The listing builds one solid part. Answer for the finished solid, in the listing's coordinates (mm). A direction names the side the tool comes from. Coordinates: 2 decimals unless noted, no trailing zeros. Loops run counter-clockwise (first coordinate to the right, second up) from the corner with the lowest first, then second, coordinate; pieces in that order, holes last. Notation, with made-up numbers: (70, -30) -> (82, -30) arc R27 ccw to (82, -1) -> close; hole circle Ø4 at (72.5, -19). An arc over 180 degrees is marked (long way). Answer in a Markdown table with one row per item.
Autodesk Inventor part; units mm, degrees
ref_plane "YZ Plane" through (0, 0, 0) normal (1, 0, 0) x (0, 1, 0)
ref_plane "XZ Plane" through (0, 0, 0) normal (0, 1, 0) x (-1, 0, 0)
ref_plane "XY Plane" through (0, 0, 0) normal (0, 0, 1) x (1, 0, 0)
sketch "Sketch1" plane through (0, 0, 0) normal (0, 0, 1) x (1, 0, 0)
  line L0 (0, 0) -> (-156.093, 0)
  line L1 (0, 162.7083) -> (0, 161.1083)
  line L2 (0, 162.7083) -> (-11.5803, 177.8)
  line L3 (-11.5803, 177.8) -> (-53.9, 177.8)
  line L4 (-53.9, 177.8) -> (-88.6, 212.5)
  line L5 (-88.6, 212.5) -> (-88.6, 292.5)
  line L6 (-88.6, 292.5) -> (-141, 292.5)
  line L7 (-141, 292.5) -> (-141, 212.5)
  line L8 (-141, 212.5) -> (-143, 212.5)
  line L9 (-143, 212.5) -> (-143, 161.1083)
  line L10 (-143, 161.1083) -> (0, 161.1083)
  dimension "d0" = 37.5
  dimension "d2" = 2
  dimension "d3" = 52.4
  dimension "d4" = 585
  dimension "d5" = 322.2165
  dimension "d7" = 425
  dimension "d8" = 1.6
  dimension "d9" = 425
  dimension "d10" = 45
  dimension "d11" = 355.6
  dimension "d24" = 141
revolve "Revolution1" add sketch "Sketch1" angle 360 about axis through (0, 0, 0) along (-1, 0, 0)
sketch "Sketch2" plane through (-88.6, 0, 0) normal (1, 0, 0) x (0, 0, -1)
  point P0 (0, 0)
  point P1 (0, 257.2)
  dimension "d13" = 257.2
hole "Hole1" at (-88.6, 257.2, 0) direction (-1, 0, 0) diameter 31.75 end up to surface
pattern_circular "Circular Pattern1" count 20 over 360 about axis through (-71.5, 0, 0) along (1, 0, 0) of "Hole1"
properties part number "Weldneck Flange 14 in" material "ASTM A105 Gr.B"
Item 1: A tool of negligible diameter and unlimited length cuts with its end or side. For faces 4 (the face through (-141, -153, -153)), 5 (the face through (-115.17, -4.77, 242.06)), from which of +Z, -Z, +X, -X, +Y, -Y can it reach the whole face along a straight path? Write none if from no direction.
Findings below:
| item | result |
|---|---|
| face 4 | -X |
| face 5 | +X, -X |
Item 2: A cutting plane is placed at A-A, the plane z = 0. Determine the outline of the cut face in (x, y) (3 decimals).
Findings below:
| item | result |
|---|---|
| outline | (-143, -212.5) -> (-141, -212.5) -> (-141, -241.325) -> (-88.6, -241.325) -> (-88.6, -212.5) -> (-53.9, -177.8) -> (-11.58, -177.8) -> (0, -162.708) -> (0, -161.108) -> (-143, -161.108) -> close; (-143, 161.108) -> (0, 161.108) -> (0, 162.708) -> (-11.58, 177.8) -> (-53.9, 177.8) -> (-88.6, 212.5) -> (-88.6, 241.325) -> (-141, 241.325) -> (-141, 212.5) -> (-143, 212.5) -> close; (-141, -292.5) -> (-88.6, -292.5) -> (-88.6, -273.075) -> (-141, -273.075) -> close; (-141, 273.075) -> (-88.6, 273.075) -> (-88.6, 292.5) -> (-141, 292.5) -> close |
Item 3: A cutting plane is placed at B-B, the plane x = -110. Count the separate pieces of the cut face and the enclosed holes in it, plus the area to 3 significant figures.
Findings below:
| item | result |
|---|---|
| separate pieces | 1 |
| enclosed holes | 21 |
| area | 171,000 mm2 |
Item 4: Find the intervals of material crossed by probe 1 along Z at (x, y) = (-91, 216.5); probe 2 along Y at (x, z) = (-102, -66); probe 3 along X at (y, z) = (172, -149), in increasing order.
Findings below:
| item | result |
|---|---|
| probe 1 | z = -196.68 to -164.64, -137.72 to 137.72, 164.64 to 196.68 |
| probe 2 | y = -284.96 to -253, -236.23 to -146.97, 146.97 to 236.23, 253 to 284.96 |
| probe 3 | x = -141 to -88.6 |
Item 5: Flat-ended cylindrical pins translate along their axes: pin 1 Ø19 at (y, z) = (0, 257.2) entering from -X; pin 2 Ø6 at (x, y) = (-58.5, -77) entering from +Z; pin 3 Ø4 at (y, z) = (117.5, -197) entering from -X; pin 4 Ø8 at (x, y) = (-120.5, -142.5) entering from -Z. Find the tip coordinate at first contact, or state that the pin passes through.
Findings below:
| item | result |
|---|---|
| pin 1 | passes through |
| pin 2 | stops at z = 168.92 |
| pin 3 | stops at x = -141 |
| pin 4 | stops at z = -257.63 |
Item 6: A cutting plane is placed at C-C, the plane x = -66. Determine the outline of the cut face in (y, z), plus the area to 3 significant figures.
Findings below:
| item | result |
|---|---|
| outline | circle Ø379.8 at (0, 0); hole circle Ø322.22 at (0, 0) |
| area | 31,700 mm2 |
Item 7: Determine the mould class of faces 1 (the face through (-33.04, 169.59, -53.41)), 2 (the face through (-115.17, -4.77, -272.34)), 3 (the face through (-143, -32.5, -158.4)) for opening direction Z: +Z half, -Z half, draft (parallel to the pull), parting line (faces both ways), or undercut.
Findings below:
| item | result |
|---|---|
| face 1 | parting line |
| face 2 | undercut |
| face 3 | draft |
